Input: part model. Units: mm. Frame: model coordinates. Coordinates: 2 decimals unless noted, no trailing zeros. Write each loop counter-clockwise with the first axis right and the second up, starting at its lowest first coordinate (ties: lowest second). Pieces come first, ordered by that corner, then holes.
1) Section query B-B (y = -3.75). Output: boundary loops of the cut face in (x, z), then the cut area to 3 significant figures.
2) Draft query along X for faces 1 (the flat face through (-1, -4, 0)), 2 (the flat face through (-37.5, -4, 19)), 3 (the cylindrical face through (-25.05, -4.06, 30.7)). Return one class per face: pulls with the +X half, pulls with the -X half, needs draft (parallel to the pull), parting line crosses it, or undercut.
3) Section query A-A (z = 28). Output: boundary loops of the cut face in (x, y).
4) Line query: L1, parallel to X at y = -7, z = 29.5; L2, parallel to Z at x = 28, y = -3.5; L3, parallel to X at y = -6.25, z = 26. Output: solid intervals per line, ascending.
5) Section query C-C (x = -28). Output: boundary loops of the cut face in (y, z), then the cut area to 3 significant figures.
from build123d import *

# Parameters (mm, degrees)
SKETCH1_W               = 75
SKETCH1_H               = 8
BOSS_EXTRUDE1_DEPTH     = 38
CUT_EXTRUDE1_DEPTH      = 54.983793864
CUT_EXTRUDE1_DEPTH_BACK = 54.983793864
SKETCH2_R               = 4


with BuildPart() as part:
    # Sketch1 → Boss-Extrude1 (new body)
    with BuildSketch(Plane.XY):
        with Locations((0, -4)):
            Rectangle(SKETCH1_W, SKETCH1_H)
    extrude(amount=BOSS_EXTRUDE1_DEPTH)

    # Sketch2 → Cut-Extrude1 (cut, two sides: drawn at the far end of the back side and taken through both)
    with BuildSketch(Plane(origin=(0, 0, 0), x_dir=(1, 0, 0), z_dir=(0, 1, 0)).offset(-CUT_EXTRUDE1_DEPTH_BACK)):
        with Locations(Location((-28, -28, 0), (0, 0, 180))):
            Circle(SKETCH2_R)
        with Locations((28, -28)):
            Circle(SKETCH2_R)
    extrude(amount=CUT_EXTRUDE1_DEPTH + CUT_EXTRUDE1_DEPTH_BACK, mode=Mode.SUBTRACT)


solid = part.part
Answer:
1. outline: (-37.5, 0) - (37.5, 0) - (37.5, 38) - (-37.5, 38) - close; hole circle Ø8 at (-28, 28); hole circle Ø8 at (28, 28)
1. area: 2,750 mm2
2. face 1: needs draft
2. face 2: pulls with the -X half
2. face 3: undercut
3. outline: (-37.5, -8) - (-32, -8) - (-32, 0) - (-37.5, 0) - close; (-24, -8) - (24, -8) - (24, 0) - (-24, 0) - close; (32, -8) - (37.5, -8) - (37.5, 0) - (32, 0) - close
4. L1: x = -37.5 to -31.71, -24.29 to 24.29, 31.71 to 37.5
4. L2: z = 0 to 24, 32 to 38
4. L3: x = -37.5 to -31.46, -24.54 to 24.54, 31.46 to 37.5
5. outline: (-8, 0) - (0, 0) - (0, 24) - (-8, 24) - close; (-8, 32) - (0, 32) - (0, 38) - (-8, 38) - close
5. area: 240 mm2
